Source: three-view drawing plus pictorial views. Frame: mm from the lowest corner of the part. A direction names the side the tool comes from. Give positions to 0.01 mm unless a question says otherwise; leave off trailing zeros. Order: outer loops, then holes, each group sorted by start corner. A loop starts at its lowest first (then second) coordinate and runs counter-clockwise, first axis right, second up. Notation, with made-up numbers: M 30.25,71.25 L 59.25,71.25 A32 ccw 59.25,109.25 Z; hole C 36,70 d1. An arc over 180 degrees is marked long. Use CSV: the item, a comma, the result in double quotes.
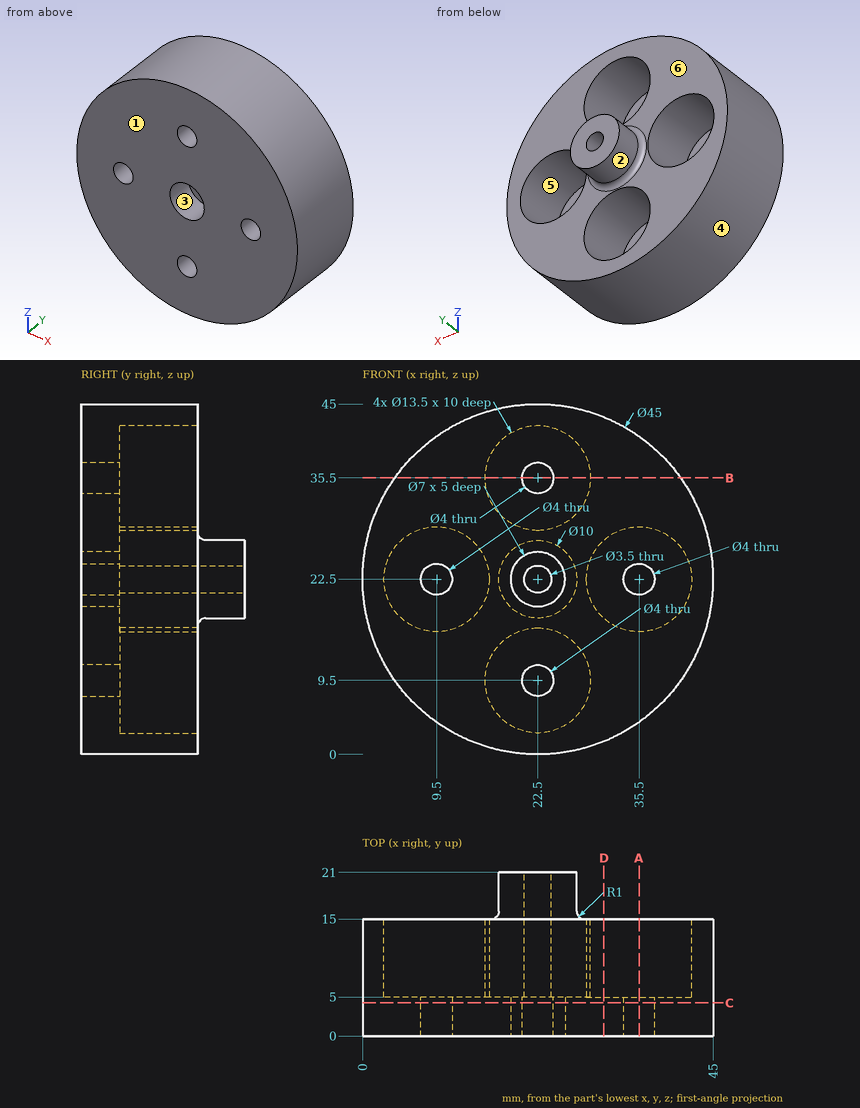
1. Pull-direction query (Z, two-part tool) for the marked faces 4, 5 and 6; classes: +Z half, -Z half, draft (parallel to the pull), parting line (faces both ways), or undercut.
Answer:
face 4,"parting line"
face 5,"undercut"
face 6,"draft"
2. Section C-C, the plane y = 4.25. Return the cut outline in (x, z), plus the area to 3 significant figures.
Answer:
outline,"C 22.5,22.5 d45; hole C 9.5,22.5 d4; hole C 22.5,22.5 d7; hole C 22.5,9.5 d4; hole C 22.5,35.5 d4; hole C 35.5,22.5 d4"
area,"1,500 mm2"
3. Section A-A, the plane x = 35.5. Return the cut outline in (y, z), plus the area to 3 significant figures.
Answer:
outline,"M 0,4.14 L 15,4.14 L 15,15.75 L 5,15.75 L 5,20.5 L 0,20.5 Z; M 0,24.5 L 5,24.5 L 5,29.25 L 15,29.25 L 15,40.86 L 0,40.86 Z"
area,"396 mm2"
4. Section D-D, the plane x = 31. Return the cut outline in (y, z).
Answer:
outline,"M 0,1.67 L 15,1.67 L 15,17.47 L 5,17.47 L 5,27.53 L 15,27.53 L 15,43.33 L 0,43.33 Z"
5. Line query: line 1 (X direction, y = 14, z = 23); line 2 (Z direction, x = 27, y = 12.5); line 3 (X direction, y = 1.75, z = 23.5). Output: solid intervals per line, ascending.
Answer:
line 1,"0.01 to 2.77, 16.23 to 20.82, 24.18 to 28.77, 42.23 to 44.99"
line 2,"0.45 to 4.47, 14.53 to 30.47, 40.53 to 44.55"
line 3,"0.02 to 7.77, 11.23 to 19.15, 25.85 to 33.77, 37.23 to 44.98"
6. Section B-B, the plane z = 35.5. Return the cut outline in (x, y).
Answer:
outline,"M 4.14,0 L 20.5,0 L 20.5,5 L 15.75,5 L 15.75,15 L 4.14,15 Z; M 24.5,0 L 40.86,0 L 40.86,15 L 29.25,15 L 29.25,5 L 24.5,5 Z"
7. Reachability of the marked faces 1, 2 and 3 from +Z, -Z, +X, -X, +Y, -Y: full face, straight path, thin tool, end or side. Return the list, or none.
Answer:
face 1,"+Z, -Z, +X, -X, -Y"
face 2,"+Y"
face 3,"-Y"
8. Pin query (flat end, axial travel): pin 1 Ø3 at (x, z) = (9.5, 22.5) entering from +Y (3 decimals); pin 2 Ø11 at (x, z) = (10, 21.5) entering from +Y; pin 3 Ø5 at (y, z) = (14.5, 27) entering from +X; pin 4 Ø21.5 at (x, z) = (9.5, 22.5) entering from +Y. Return the tip coordinate at first contact, or that it passes through.
Answer:
pin 1,"through"
pin 2,"y = 5"
pin 3,"x = 44.91"
pin 4,"y = 21"
